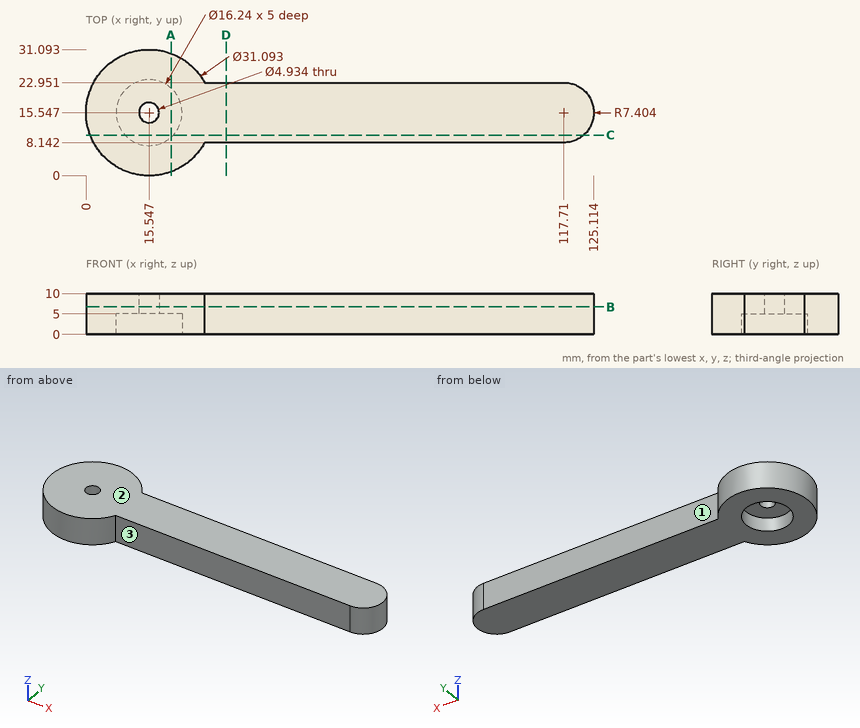
Could you check a few things on this drawing? It's one solid part, dimensions in mm from its lowest x, y, z. A direction names the side the tool comes from. Coordinates: 2 decimals unless noted, no trailing zeros. Write each loop counter-clockwise with the first axis right and the second up, starting at its lowest first coordinate (ties: lowest second). Pieces come first, ordered by that corner, then holes.
Q1. For P1, Ø5, axis at x = 73, z = 2.5, coming from the +Y side; P2, Ø1.5, axis at x = 62.5, z = 6.5, coming from the -Y side; P3, Ø4.5, axis at x = 15.55, y = 15.55, coming from the +Z side; P4, Ø3, axis at x = 25, z = 1.5, coming from the +Y side (1 decimal), each with a flat end and sliding along its axis, tell me the tip position at first contact or that it passes through.
Results found:
P1: stops at y = 22.95
P2: stops at y = 8.14
P3: passes through
P4: stops at y = 28.9
Q2. Please list where these lines run through material, in increasing order: L1, parallel to X at y = 15, z = 4 (1 decimal); L2, parallel to Y at x = 83, z = 4.75; L3, parallel to Y at x = 16, z = 8.
Results found:
L1: x = 0 to 7.4, 23.6 to 125.1
L2: y = 8.14 to 22.95
L3: y = 0.01 to 13.12, 17.97 to 31.09
Q3. Imagine slicing it at C-C, the plane y = 10. List the corners of the cut face in (x, z) for me (1 decimal), plus the area to 3 significant figures.
Results found:
outline: (1, 0) - (9.6, 0) - (9.6, 5) - (21.5, 5) - (21.5, 0) - (122.6, 0) - (122.6, 10) - (1, 10) - close
area: 1,160 mm2
Q4. Imagine slicing it at B-B, the plane z = 6.75. List the corners of the cut face in (x, y) for me (1 decimal), plus the area to 3 significant figures.
Results found:
outline: (29.2, 8.1) - (117.7, 8.1) arc R7.4 ccw to (117.7, 23) - (29.2, 23) arc R15.5 ccw (long way) to start; hole circle Ø4.9 at (15.5, 15.5)
area: 2,120 mm2
Q5. Imagine slicing it at A-A, the plane x = 21. List the corners of the cut face in (y, z) for me (1 decimal).
Results found:
outline: (1, 0) - (9.5, 0) - (9.5, 5) - (21.6, 5) - (21.6, 0) - (30.1, 0) - (30.1, 10) - (1, 10) - close
Q6. Which directions (+Z, -Z, +X, -X, +Y, -Y) give clear straight access to the entire face, cutting with the end or side of a thin tool? Please do the marked faces 1, 2 and 3.
Results found:
face 1: +Z, -Z, +X, +Y
face 2: +Z, +X, -X, +Y, -Y
face 3: +Z, -Z, +X, -Y
Q7. Imagine slicing it at D-D, the plane x = 34.5. List the corners of the cut face in (y, z) for me.
Results found:
outline: (8.14, 0) - (22.95, 0) - (22.95, 10) - (8.14, 10) - close
